from build123d import *

# Parameters (mm, degrees)
SKETCH_1_R      = 1.6
EXTRUDE_1_DEPTH = 3
EXTRUDE_2_DEPTH = 3
FILLET_1_R      = 2
FILLET_2_R      = 2


with BuildPart() as part:
    # 草图1 → 凸台-拉伸1 (new body)
    with BuildSketch(Plane(origin=(0, 0, 0), x_dir=(1, 0, 0), z_dir=(0, 1, 0))):
        Polygon((-14.5, -4), (-14.5, 4), (12.5, 4), (12.5, 8), (18.5, 8), (18.5, 5), (16, 5), (16, -5), (18.5, -5), (18.5, -8), (12.5, -8), (12.5, -4), align=None)
        with Locations(Location((11, 0, 0), (0, 0, 270))):
            Circle(SKETCH_1_R, mode=Mode.SUBTRACT)
    extrude(amount=EXTRUDE_1_DEPTH)

    # 草图3 → 凸台-拉伸2 (add)
    with BuildSketch(Plane.ZY.offset(14.5)):
        with BuildLine():
            Line((-4, 15), (-4, 3))
            Line((-4, 3), (4, 3))
            Line((4, 3), (4, 15))
            ThreePointArc((4, 15), (3.69551813, 16.530733729), (2.828427125, 17.828427125))
            Line((2.828427125, 17.828427125), (1.272792206, 16.272792206))
            ThreePointArc((1.272792206, 16.272792206), (0, 13.2), (-1.272792206, 16.272792206))
            Line((-1.272792206, 16.272792206), (-2.828427125, 17.828427125))
            ThreePointArc((-2.828427125, 17.828427125), (-3.69551813, 16.530733729), (-4, 15))
        make_face()
    extrude(amount=-EXTRUDE_2_DEPTH)

    # 圆角1
    fillet_1_edges = [part.edges().sort_by_distance(p)[0] for p in [
        (12.5, 1.5, -8),
        (18.5, 1.5, -8),
        (18.5, 1.5, 8),
        (12.5, 1.5, 8),
    ]]
    fillet(fillet_1_edges, radius=FILLET_1_R)

    # 圆角2
    fillet_2_edges = [part.edges().sort_by_distance(p)[0] for p in [
        (-14.5, 0, 0),
        (-11.5, 3, 0),
    ]]
    fillet(fillet_2_edges, radius=FILLET_2_R)


solid = part.part
The model under review builds one solid part; all positions refer to its coordinate system, in mm. A direction names the side the tool comes from. Round coordinates to 2 decimals unless told otherwise and drop trailing zeros. Loops run counter-clockwise (first coordinate to the right, second up) from the corner with the lowest first, then second, coordinate; pieces in that order, holes last. Notation, with made-up numbers: (56.5, -25.75) -> (89.5, -25.75) arc R16 ccw to (89.5, -21.75) -> close; hole circle Ø10 at (-19.5, 57.5). An arc over 180 degrees is marked (long way). One line per question, with ' | ' between items. Start each with the question number.
Item 1: Add section C-C, the plane y = 7.5. Write out the cut boundary in (x, z), then the cut area to 3 significant figures.
Item 2: Wall thickness on line 1 along X through (y, z) = (1.9, 0); line 2 along Y through (x, z) = (-12.6, 0); line 3 along X through (y, z) = (11.75, -2.25): over which ranges is each line inside the solid? List them lowest first. Write a range as [from, to].
Item 3: Add section B-B, the plane x = -6. Write out the cut boundary in (y, z).
Item 4: Add section A-A, the plane z = 0. Write out the cut boundary in (x, y).
Item 5: Machinability: for faces 1 (the face through (12.5, 1, 5)), 2 (the face through (-13, 17, -2)), 3 (the face through (-5.1, 2.5, -4)), which of the approach directions +Z, -Z, +X, -X, +Y, -Y give a long, thin tool a straight path to every point of the face, cutting with its end or side? Answer none if there is none.
Item 6: For pin 1 (3 mm diameter, centred on x = 11, z = 0, fed in from -Y); pin 2 (2.5 mm diameter, centred on y = 1.5, z = -1, fed in from +X); pin 3 (0.6 mm diameter, centred on y = 1.5, z = -5, fed in from -X); pin 4 (4 mm diameter, centred on y = 10.5, z = -1.5, fed in from +X), all flat-tipped, find the tip position at first contact; note any pin that passes through.
Item 7: Draft analysis for pull direction Z (two halves, no side actions). For faces 4 (the face through (-13.021, 16.551, -3.687)), 5 (the face through (5, 3, 0)), 6 (the face through (-13, 17, 2)), 7 (the face through (16, 1, 0)), state which applies: +Z half, -Z half, draft (parallel to the pull), parting line (faces both ways), or undercut.
Return value:
1) outline: (-14.5, -4) -> (-11.5, -4) -> (-11.5, 4) -> (-14.5, 4) -> close | area: 24.0 mm2
2) line 1: x = [-14.5, 9.4], [12.6, 16] | line 2: y = [0, 13.2] | line 3: x = [-14.5, -11.5]
3) outline: (0, -4) -> (3, -4) -> (3, 4) -> (0, 4) -> close
4) outline: (-14.5, 2) arc R2 ccw to (-12.5, 0) -> (9.4, 0) -> (9.4, 3) -> (-9.5, 3) arc R2 cw to (-11.5, 5) -> (-11.5, 13.2) -> (-14.5, 13.2) -> close; (12.6, 0) -> (16, 0) -> (16, 3) -> (12.6, 3) -> close
5) face 1: +Z, -X, +Y, -Y | face 2: +X, -X, +Y | face 3: -Z, -X, +Y, -Y
6) pin 1: passes through | pin 2: stops at x = 16 | pin 3: stops at x = 12.5 | pin 4: stops at x = -11.5
7) face 4: -Z half | face 5: draft | face 6: undercut | face 7: undercut
